from build123d import *

# Parameters (mm, degrees)
SKETCH1_W           = 95
SKETCH1_H           = 33
BOSS_EXTRUDE1_DEPTH = 18
SKETCH2_W           = 10.831848702
SKETCH2_H           = 22.331730537
BOSS_EXTRUDE2_DEPTH = 10
FILLET1_R           = 3


with BuildPart() as part:
    # Sketch1 → Boss-Extrude1 (new body)
    with BuildSketch(Plane(origin=(0, 0, 0), x_dir=(0, 0, -1), z_dir=(1, 0, 0))):
        Rectangle(SKETCH1_W, SKETCH1_H)
    extrude(amount=BOSS_EXTRUDE1_DEPTH)

    # Sketch2 → Boss-Extrude2 (add)
    with BuildSketch(Plane.XY.offset(47.5)):
        with Locations((8.498326505, 1.139612194)):
            Rectangle(SKETCH2_W, SKETCH2_H)
    extrude(amount=BOSS_EXTRUDE2_DEPTH)

    # Fillet1
    fillet1_edges = [part.edges().sort_by_distance(p)[0] for p in [
        (18, -16.5, 0),
        (0, -16.5, 0),
        (0, 16.5, 0),
        (18, 16.5, 0),
    ]]
    fillet(fillet1_edges, radius=FILLET1_R)


solid = part.part
The listing builds one solid part. Answer for the finished solid, in the listing's coordinates (mm). A direction names the side the tool comes from. Give positions to 0.01 mm unless a question says otherwise; leave off trailing zeros. Loops run counter-clockwise (first coordinate to the right, second up) from the corner with the lowest first, then second, coordinate; pieces in that order, holes last. Notation, with made-up numbers: (6, 4.25) - (39, 4.25) arc R23 cw to (39, 22.25) - close; hole circle Ø10 at (20, 11.25). An arc over 180 degrees is marked (long way). Answer as a JSON object with one key per item and string values.
1. A cutting plane is placed at A-A (y = -8). Write down the section's boundary in (x, z).
Determined:
{"outline": "(0, -47.5) - (18, -47.5) - (18, 47.5) - (13.91, 47.5) - (13.91, 57.5) - (3.08, 57.5) - (3.08, 47.5) - (0, 47.5) - close"}
2. A cutting plane is placed at B-B (x = 11.5). Write down the section's boundary in (y, z).
Determined:
{"outline": "(-16.5, -47.5) - (16.5, -47.5) - (16.5, 47.5) - (12.31, 47.5) - (12.31, 57.5) - (-10.03, 57.5) - (-10.03, 47.5) - (-16.5, 47.5) - close"}
3. For faces 1 (the flat face through (8, -10.026, 52)), 2 (the flat face through (13.914, 1, 52)), 3 (the flat face through (8, 12.305, 52)), determine the directions among +Z, -Z, +X, -X, +Y, -Y from which every point of the face is accessible in a straight line to the end or side of a thin tool.
Determined:
{"face 1": "+Z, +X, -X, -Y", "face 2": "+Z, +X, +Y, -Y", "face 3": "+Z, +X, -X, +Y"}
4. Flat-ended cylindrical pins translate along their axes: pin 1 Ø11 at (y, z) = (1, 53.5) entering from +X; pin 2 Ø3 at (x, z) = (11, 50.5) entering from -Y. Find the tip coordinate at first contact, or state that the pin passes through.
Determined:
{"pin 1": "x = 13.91", "pin 2": "y = -10.03"}
5. A cutting plane is placed at D-D (x = 16.5). Write down the section's boundary in (y, z).
Determined:
{"outline": "(-16.1, -47.5) - (16.1, -47.5) - (16.1, 47.5) - (-16.1, 47.5) - close"}
6. A cutting plane is placed at C-C (y = -12). Write down the section's boundary in (x, z), then the cut area to 3 significant figures.
Determined:
{"outline": "(0, -47.5) - (18, -47.5) - (18, 47.5) - (0, 47.5) - close", "area": "1,710 mm²"}
7. Find the intervals of material crossed by L1, parallel to Z at x = 8.5, y = 14; L2, parallel to Y at x = 15.75, z = 24.5; L3, parallel to X at y = 15, z = 34, in increasing order. Write a range as [from, to].
Determined:
{"L1": "[-47.5, 47.5]", "L2": "[-16.4, 16.4]", "L3": "[0.4, 17.6]"}
